Geometry check sheet. Reference: drawing and pictorial views, mm from the part's lowest x, y, z. Coordinates: 2 decimals unless noted, no trailing zeros. Loops run counter-clockwise (first coordinate to the right, second up) from the corner with the lowest first, then second, coordinate; pieces in that order, holes last. Notation, with made-up numbers: (52, 75) -> (107, 75) arc R17 cw to (107, 97) -> close; hole circle Ø9 at (-32.5, 51). An arc over 180 degrees is marked (long way). Use CSV: the item, a comma, the result in double quotes.
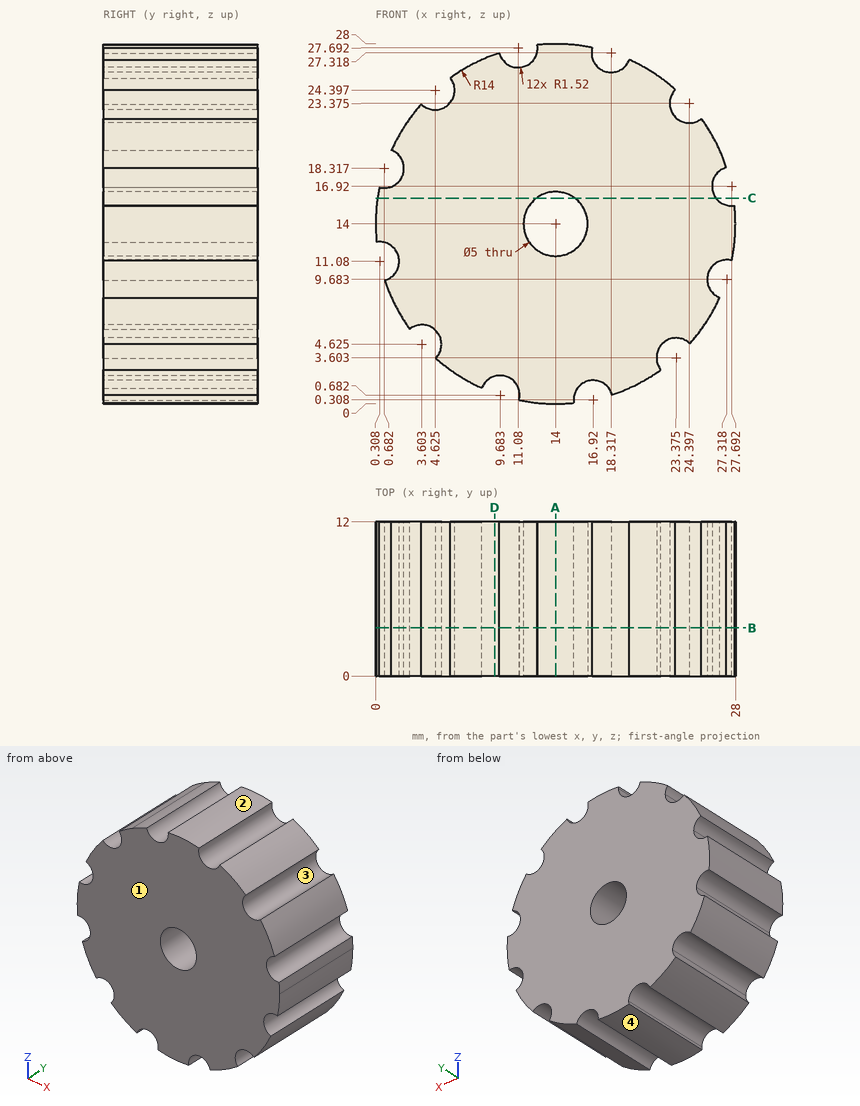
1) Cross-section at C-C on z = 16. Record the boundary of the cut face in (x, y), and give its area (3 significant figures).
Answer below:
outline,"(0.14, 0) -> (12.5, 0) -> (12.5, 12) -> (0.14, 12) -> close; (15.5, 0) -> (26.48, 0) -> (26.48, 12) -> (15.5, 12) -> close"
area,"280 mm²"
2) Go/stop test with flat-tipped pins: pin 1 Ø1.5 at (y, z) = (10.5, 4.5) entering from -X (1 decimal); pin 2 Ø1 at (y, z) = (5.5, 21) entering from +X; pin 3 Ø4 at (x, y) = (3.5, 9) entering from -Z (1 decimal). Record where each tip stops, or that it passes through.
Answer below:
pin 1,"stops at x = 4.8"
pin 2,"stops at x = 26.4"
pin 3,"stops at z = 2.9"
3) Cross-section at B-B on y = 3.75. Record the boundary of the cut face in (x, z) (1 decimal).
Answer below:
outline,"(0.1, 12.6) arc R1.5 cw to (0.7, 9.6) arc R14 ccw to (2.6, 5.8) arc R1.5 cw to (4.7, 3.6) arc R14 ccw to (8.3, 1.2) arc R1.5 cw to (11.2, 0.3) arc R14 ccw to (15.4, 0.1) arc R1.5 cw to (18.4, 0.7) arc R14 ccw to (22.2, 2.6) arc R1.5 cw to (24.4, 4.7) arc R14 ccw to (26.8, 8.3) arc R1.5 cw to (27.7, 11.2) arc R14 ccw to (27.9, 15.4) arc R1.5 cw to (27.3, 18.4) arc R14 ccw to (25.4, 22.2) arc R1.5 cw to (23.3, 24.4) arc R14 ccw to (19.7, 26.8) arc R1.5 cw to (16.8, 27.7) arc R14 ccw to (12.6, 27.9) arc R1.5 cw to (9.6, 27.3) arc R14 ccw to (5.8, 25.4) arc R1.5 cw to (3.6, 23.3) arc R14 ccw to (1.2, 19.7) arc R1.5 cw to (0.3, 16.8) arc R14 ccw to start; hole circle Ø5 at (14, 14)"
4) Draft check along Z on the marked faces 1, 2, 3 and 4. Enter one of: released by +Z, released by -Z, zero draft, split by the parting line, or undercut.
Answer below:
face 1,"zero draft"
face 2,"released by +Z"
face 3,"undercut"
face 4,"released by -Z"
5) Cross-section at A-A on x = 14. Record the boundary of the cut face in (y, z).
Answer below:
outline,"(0, 0) -> (12, 0) -> (12, 11.5) -> (0, 11.5) -> close; (0, 16.5) -> (12, 16.5) -> (12, 28) -> (0, 28) -> close"
6) Cross-section at D-D on x = 9.25. Record the boundary of the cut face in (y, z), and give its area (3 significant figures).
Answer below:
outline,"(0, 2.14) -> (12, 2.14) -> (12, 27.17) -> (0, 27.17) -> close"
area,"300 mm²"
7) Thickness scan on line 1 along X through (y, z) = (8.25, 14); line 2 along Z through (x, y) = (26.5, 2.5) (1 decimal). Record the ranges inside material, lowest first. Write a range as from..to.
Answer below:
line 1,"x = 0..11.5, 16.5..28"
line 2,"z = 7.7..8.4, 11..16, 17.9..20.3"
